Geometry check sheet. Reference: the model listing, model coordinates, mm. Face numbers are marked on the shaded views. A direction names the side the tool comes from. Coordinates: 2 decimals unless noted, no trailing zeros. Write each loop counter-clockwise with the first axis right and the second up, starting at its lowest first coordinate (ties: lowest second). Pieces come first, ordered by that corner, then holes. Notation, with made-up numbers: (52, 51) -> (86, 51) arc R32 ccw to (86, 86) -> close; hole circle Ø8 at (74.5, 61). An arc over 180 degrees is marked (long way). Answer in a Markdown table with one row per item. Add a question column.
1. Mould release check, pull along Y, two halves, no side actions. Record for the marked faces 6, 7 and 8: pulls with the +Y half, pulls with the -Y half, needs draft (parallel to the pull), parting line crosses it, or undercut.
2. Cross-section at C-C on x = 23. Record the cut outline in (y, z), and give its area (3 significant figures).
3. Cross-section at A-A on z = 2.25. Record the cut outline in (x, y).
4. Cross-section at D-D on x = 8. Record the cut outline in (y, z), and give its area (3 significant figures).
5. Scan lines: L1, parallel to X at y = -10, z = 11; L2, parallel to Y at x = 0, z = 3.5; L3, parallel to Z at x = 26, y = -4.5. Record each from-to range of solid material in increasing order. Write a range as from..to.
6. Cross-section at B-B on y = 3. Record the cut outline in (x, z), and give its area (3 significant figures).
7. Set-up check for the marked faces 1, 2, 3, 4 and 5: record each of +Z, -Z, +X, -X, +Y, -Y from which the full face is reachable in a straight line by a thin tool's end or side.
8. Depth check by flat-ended pin: P1, Ø1.5, axis at x = 19.5, y = -7.5, coming from the +Z side; P2, Ø12, axis at x = -3, y = -6.5, coming from the -Z side; P3, Ø3, axis at y = 4, z = 8.5, coming from the -X side; P4, Ø5, axis at x = 23.5, z = 9, coming from the +Y side. Enter the tip coordinate at first touch or a pass-through.
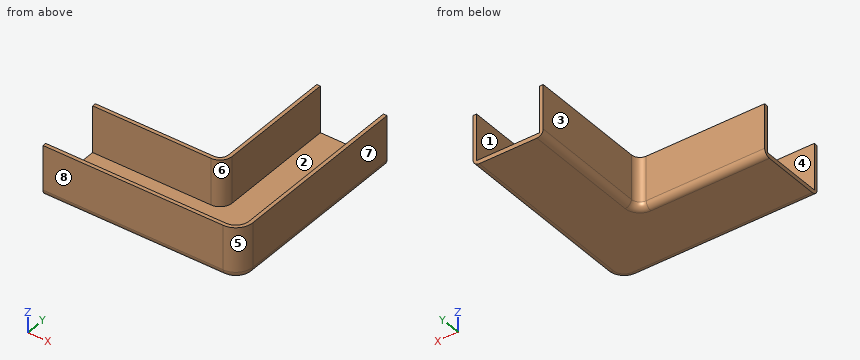
Solid Edge part; units mm, degrees
sketch "Sketch1" plane through (0, 0, 0) normal (0, 0, 1) x (1, 0, 0)
  line L0 (27.6, -31.6) -> (-15, -31.6)
  line L1 (-15, -31.6) -> (-15, -15)
  line L2 (-15, -15) -> (13, -15)
  arc A0 (15, -13) -> (13, -15) centre (13, -13) cw
  line L3 (15, -13) -> (15, 15)
  line L4 (15, 15) -> (31.6, 15)
  line L5 (31.6, 15) -> (31.6, -27.6)
  arc A1 (31.6, -27.6) -> (27.6, -31.6) centre (27.6, -27.6) cw
extrude "Protrusion1" add sketch "Sketch1" along normal blind 12
fillet "Rotondo_1" radius 1.5 6 edges at (6.3, -31.6, 0) (30.4284, -30.4284, 0) (31.6, -6.3, 0) (-1, -15, 0) (14.4142, -14.4142, 0) (15, 1, 0)
sketch "Sketch2" plane through (7.5, -7.5, 12) normal (0, 0, 1) x (0, 1, 0)
  line L0 (26.8363, -8.35) -> (26.8363, -23.25)
  line L1 (26.8363, -23.25) -> (21.4, -23.25)
  line L2 (21.4, -23.25) -> (-20.1, -23.25)
  arc A0 (-20.1, -23.25) -> (-23.25, -20.1) centre (-20.1, -20.1) cw
  line L3 (-23.25, -20.1) -> (-23.25, 21.4)
  line L4 (-23.25, 21.4) -> (-23.25, 26.0258)
  line L5 (-23.25, 26.0258) -> (-8.35, 26.0258)
  line L6 (-8.35, 26.0258) -> (-8.35, 21.4)
  line L7 (-8.35, 21.4) -> (-8.35, -5.5)
  arc A1 (-8.35, -5.5) -> (-5.5, -8.35) centre (-5.5, -5.5) ccw
  line L8 (-5.5, -8.35) -> (21.4, -8.35)
  line L9 (21.4, -8.35) -> (26.8363, -8.35)
extrude "ScavoEstrusione_3" cut sketch "Sketch2" against normal blind 11
Results found:
| question | item | result |
|---|---|---|
| 1 | face 6 | undercut |
| 1 | face 7 | needs draft |
| 1 | face 8 | pulls with the -Y half |
| 2 | outline | (-31.6, 1.5) arc R1.5 ccw to (-30.1, 0) -> (15, 0) -> (15, 1) -> (-30.75, 1) -> (-30.75, 12) -> (-31.6, 12) -> close |
| 2 | area | 55.5 mm^2 |
| 3 | outline | (-15, -31.6) -> (27.6, -31.6) arc R4 ccw to (31.6, -27.6) -> (31.6, 15) -> (30.75, 15) -> (30.75, -27.6) arc R3.15 cw to (27.6, -30.75) -> (-15, -30.75) -> close; (-15, -15.85) -> (13, -15.85) arc R2.85 ccw to (15.85, -13) -> (15.85, 15) -> (15, 15) -> (15, -13) arc R2 cw to (13, -15) -> (-15, -15) -> close |
| 4 | outline | (-31.6, 1.5) arc R1.5 ccw to (-30.1, 0) -> (-16.5, 0) arc R1.5 ccw to (-15, 1.5) -> (-15, 12) -> (-15.85, 12) -> (-15.85, 1) -> (-30.75, 1) -> (-30.75, 12) -> (-31.6, 12) -> close |
| 4 | area | 34.3 mm^2 |
| 5 | L1 | x = 15..15.85, 30.75..31.6 |
| 5 | L2 | y = -31.6..-30.75, -15.85..-15 |
| 5 | L3 | z = 0..1 |
| 6 | outline | (15, 1.5) arc R1.5 ccw to (16.5, 0) -> (30.1, 0) arc R1.5 ccw to (31.6, 1.5) -> (31.6, 12) -> (30.75, 12) -> (30.75, 1) -> (15.85, 1) -> (15.85, 12) -> (15, 12) -> close |
| 6 | area | 34.3 mm^2 |
| 7 | face 1 | +Z, +Y |
| 7 | face 2 | +Z |
| 7 | face 3 | +Z, -Z, -X, +Y |
| 7 | face 4 | +Z, -X |
| 7 | face 5 | +Z, -Z, +X, -Y |
| 8 | P1 | stops at z = 1 |
| 8 | P2 | passes through |
| 8 | P3 | stops at x = 15 |
| 8 | P4 | stops at y = -30.75 |
